Input: part model. Units: mm. Frame: model coordinates. Face numbers are marked on the shaded views. A direction names the side the tool comes from. Coordinates: 2 decimals unless noted, no trailing zeros. Write each loop counter-clockwise with the first axis right and the second up, starting at its lowest first coordinate (ties: lowest second). Pieces come first, ordered by that corner, then holes. Notation, with made-up numbers: (-13.75, -28) -> (34.25, -28) arc R24 cw to (34.25, -11) -> close; hole circle Ø3 at (51, 71). An arc over 180 degrees is marked (long way). Use one line per item in the form item = value. Start each with the question number.
(1) Cut plane A-A on x = 0. Return the cut outline in (y, z).
(2) First-contact query: pin 1 (10 mm diameter, centred on y = 6.5, z = -19, fed in from -X); pin 2 (4 mm diameter, centred on x = -9, y = 0, fed in from +Z); pin 3 (12 mm diameter, centred on x = 6.5, z = -1, fed in from -Y); pin 4 (3 mm diameter, centred on x = -10.5, y = 6, fed in from -Z). Flat tips, straight axial feed; report the tip coordinate or a pass-through.
(3) Pull-direction query (Z, two-part tool) for the marked faces 1, 2 and 3; classes: released by +Z, released by -Z, zero draft, split by the parting line, or undercut.
(4) Ray query, line 1 along Z through (x, y) = (26.5, -7.25); line 2 along X through (y, z) = (-7.45, 0); line 3 along X through (y, z) = (-7, -22.5). Return the intervals inside material, ascending.
(5) Cut plane B-B on z = 0. Return the cut outline in (x, y), plus the area to 3 significant figures.
(6) Set-up query: the marked faces 4, 5, 6, 7 and 8. Return all of +Z, -Z, +X, -X, +Y, -Y with unobstructed straight access to the full face (end or side cutting, diameter ignored); none if empty.
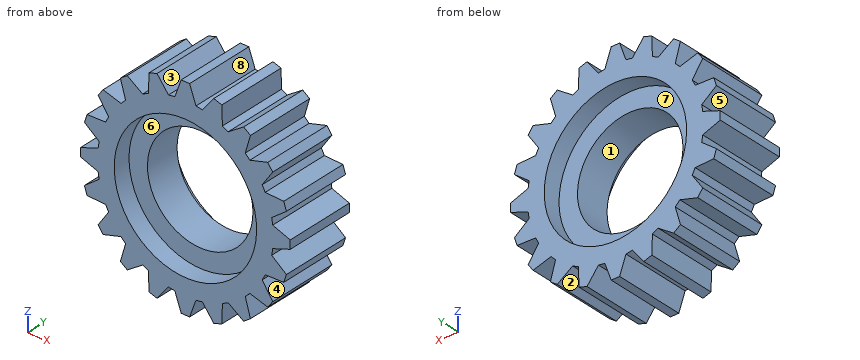
```python
from build123d import *

# Parameters (mm, degrees)
BOSS_EXTRUDE2_START     = -10
BOSS_EXTRUDE2_DEPTH     = 20
CUT_EXTRUDE1_DEPTH      = 5
CUT_EXTRUDE1_DEPTH_BACK = 5
SKETCH3_R               = 15
SKETCH4_R               = 20.25
CUT_EXTRUDE2_DEPTH      = 5


# Read off the part's stored shape, not the designer's step: Boss-Extrude2
with BuildPart() as part:
    # Boss-Extrude2 outline → Boss-Extrude2 (new body)
    with BuildSketch(Plane(origin=(0, 0, 0), x_dir=(1, 0, 0), z_dir=(0, 1, 0)).offset(BOSS_EXTRUDE2_START)):
        with BuildLine():
            Line((24.819347292, -3), (29.819347292, -1.2))
            Line((29.819347292, -1.2), (29.819347292, 1.2))
            Line((29.819347292, 1.2), (24.819347292, 3))
            ThreePointArc((24.819347292, 3), (24.692232517, 3.910710079), (24.531712075, 4.81612943))
            Line((24.531712075, 4.81612943), (28.73075389, 8.073108238))
            Line((28.73075389, 8.073108238), (27.989113104, 10.355643877))
            Line((27.989113104, 10.355643877), (22.677695772, 10.522457624))
            ThreePointArc((22.677695772, 10.522457624), (22.275365258, 11.349365736), (21.842895395, 12.160917759))
            Line((21.842895395, 12.160917759), (24.829892006, 16.555964393))
            Line((24.829892006, 16.555964393), (23.419207401, 18.497605179))
            Line((23.419207401, 18.497605179), (18.316388565, 17.014990742))
            ThreePointArc((18.316388565, 17.014990742), (17.678159939, 17.677179107), (17.016006986, 18.315444473))
            Line((17.016006986, 18.315444473), (18.498605179, 23.418207401))
            Line((18.498605179, 23.418207401), (16.556964393, 24.828892006))
            Line((16.556964393, 24.828892006), (12.162276227, 21.84213902))
            ThreePointArc((12.162276227, 21.84213902), (11.350541159, 22.274766338), (10.523440542, 22.677239672))
            Line((10.523440542, 22.677239672), (10.356643877, 27.988113104))
            Line((10.356643877, 27.988113104), (8.074108238, 28.72975389))
            Line((8.074108238, 28.72975389), (4.817670386, 24.5314095))
            ThreePointArc((4.817670386, 24.5314095), (3.911818446, 24.69205695), (3.00066912, 24.819266404))
            Line((3.00066912, 24.819266404), (1.201, 29.818347292))
            Line((1.201, 29.818347292), (-1.199, 29.818347292))
            Line((-1.199, 29.818347292), (-2.998578144, 24.819519115))
            ThreePointArc((-2.998578144, 24.819519115), (-3.909904803, 24.692360042), (-4.815934726, 24.531750299))
            Line((-4.815934726, 24.531750299), (-8.072108238, 28.72975389))
            Line((-8.072108238, 28.72975389), (-10.354643877, 27.988113104))
            Line((-10.354643877, 27.988113104), (-10.521410966, 22.678181393))
            ThreePointArc((-10.521410966, 22.678181393), (-11.348983821, 22.275559841), (-12.16117688, 21.842751129))
            Line((-12.16117688, 21.842751129), (-16.554964393, 24.828892006))
            Line((-16.554964393, 24.828892006), (-18.496605179, 23.418207401))
            Line((-18.496605179, 23.418207401), (-17.014432073, 18.316907524))
            ThreePointArc((-17.014432073, 18.316907524), (-17.677179115, 17.678159931), (-18.315963478, 17.01544833))
            Line((-18.315963478, 17.01544833), (-23.417207401, 18.497605179))
            Line((-23.417207401, 18.497605179), (-24.827892006, 16.555964393))
            Line((-24.827892006, 16.555964393), (-21.841994742, 12.162535331))
            ThreePointArc((-21.841994742, 12.162535331), (-22.274960948, 11.350159239), (-22.677725349, 10.522393882))
            Line((-22.677725349, 10.522393882), (-27.987113104, 10.355643877))
            Line((-27.987113104, 10.355643877), (-28.72875389, 8.073108238))
            Line((-28.72875389, 8.073108238), (-24.531447735, 4.817475691))
            ThreePointArc((-24.531447735, 4.817475691), (-24.692184512, 3.91101317), (-24.819438268, 2.999247249))
            Line((-24.819438268, 2.999247249), (-29.817347292, 1.2))
            Line((-29.817347292, 1.2), (-29.817347292, -1.2))
            Line((-29.817347292, -1.2), (-24.819438268, -2.999247249))
            ThreePointArc((-24.819438268, -2.999247249), (-24.692184512, -3.91101317), (-24.531447735, -4.817475691))
            Line((-24.531447735, -4.817475691), (-28.72875389, -8.073108238))
            Line((-28.72875389, -8.073108238), (-27.987113104, -10.355643877))
            Line((-27.987113104, -10.355643877), (-22.677725349, -10.522393882))
            ThreePointArc((-22.677725349, -10.522393882), (-22.274960948, -11.350159239), (-21.841994742, -12.162535331))
            Line((-21.841994742, -12.162535331), (-24.827892006, -16.555964393))
            Line((-24.827892006, -16.555964393), (-23.417207401, -18.497605179))
            Line((-23.417207401, -18.497605179), (-18.315963478, -17.01544833))
            ThreePointArc((-18.315963478, -17.01544833), (-17.677179115, -17.678159931), (-17.014432073, -18.316907524))
            Line((-17.014432073, -18.316907524), (-18.496605179, -23.418207401))
            Line((-18.496605179, -23.418207401), (-16.554964393, -24.828892006))
            Line((-16.554964393, -24.828892006), (-12.16117688, -21.842751129))
            ThreePointArc((-12.16117688, -21.842751129), (-11.348983821, -22.275559841), (-10.521410966, -22.678181393))
            Line((-10.521410966, -22.678181393), (-10.354643877, -27.988113104))
            Line((-10.354643877, -27.988113104), (-8.072108238, -28.72975389))
            Line((-8.072108238, -28.72975389), (-4.815934726, -24.531750299))
            ThreePointArc((-4.815934726, -24.531750299), (-3.909904803, -24.692360042), (-2.998578144, -24.819519115))
            Line((-2.998578144, -24.819519115), (-1.199, -29.818347292))
            Line((-1.199, -29.818347292), (1.201, -29.818347292))
            Line((1.201, -29.818347292), (3.00066912, -24.819266404))
            ThreePointArc((3.00066912, -24.819266404), (3.911818446, -24.69205695), (4.817670386, -24.5314095))
            Line((4.817670386, -24.5314095), (8.074108238, -28.72975389))
            Line((8.074108238, -28.72975389), (10.356643877, -27.988113104))
            Line((10.356643877, -27.988113104), (10.523440542, -22.677239672))
            ThreePointArc((10.523440542, -22.677239672), (11.350541159, -22.274766338), (12.162276227, -21.84213902))
            Line((12.162276227, -21.84213902), (16.556964393, -24.828892006))
            Line((16.556964393, -24.828892006), (18.498605179, -23.418207401))
            Line((18.498605179, -23.418207401), (17.016006986, -18.315444473))
            ThreePointArc((17.016006986, -18.315444473), (17.678159939, -17.677179107), (18.316388565, -17.014990742))
            Line((18.316388565, -17.014990742), (23.419207401, -18.497605179))
            Line((23.419207401, -18.497605179), (24.829892006, -16.555964393))
            Line((24.829892006, -16.555964393), (21.842895395, -12.160917759))
            ThreePointArc((21.842895395, -12.160917759), (22.275365258, -11.349365736), (22.677695772, -10.522457624))
            Line((22.677695772, -10.522457624), (27.989113104, -10.355643877))
            Line((27.989113104, -10.355643877), (28.73075389, -8.073108238))
            Line((28.73075389, -8.073108238), (24.531712075, -4.81612943))
            ThreePointArc((24.531712075, -4.81612943), (24.692232517, -3.910710079), (24.819347292, -3))
        make_face()
    extrude(amount=BOSS_EXTRUDE2_DEPTH)

    # Sketch3 → Cut-Extrude1 (cut, two sides: drawn at the far end of the back side and taken through both)
    with BuildSketch(Plane(origin=(0, 0, 0), x_dir=(1, 0, 0), z_dir=(0, 1, 0)).offset(-CUT_EXTRUDE1_DEPTH_BACK)):
        with Locations(Location((0, 0, 0), (0, 0, 270))):
            Circle(SKETCH3_R)
    extrude(amount=CUT_EXTRUDE1_DEPTH + CUT_EXTRUDE1_DEPTH_BACK, mode=Mode.SUBTRACT)

    # Sketch4 → Cut-Extrude2 (cut)
    with BuildSketch(Plane(origin=(0, 10, 0), x_dir=(1, 0, 0), z_dir=(0, 1, 0))):
        with Locations(Location((0, 0, 0), (0, 0, 270))):
            Circle(SKETCH4_R)
    cut_extrude2 = extrude(amount=-CUT_EXTRUDE2_DEPTH, mode=Mode.SUBTRACT)

    # Mirror1: Cut-Extrude2 across plane
    add(cut_extrude2.mirror(Plane.ZX), mode=Mode.SUBTRACT)


solid = part.part
```
Values:
q1.outline = (-10, -29.82) -> (10, -29.82) -> (10, -20.25) -> (5, -20.25) -> (5, -15) -> (-5, -15) -> (-5, -20.25) -> (-10, -20.25) -> close; (-10, 20.25) -> (-5, 20.25) -> (-5, 15) -> (5, 15) -> (5, 20.25) -> (10, 20.25) -> (10, 29.82) -> (-10, 29.82) -> close
q2.pin_1 = -24.83
q2.pin_2 = 28.73
q2.pin_3 = through
q2.pin_4 = -28.43
q3.face_1 = undercut
q3.face_2 = released by -Z
q3.face_3 = released by +Z
q4.line_1 = -10.4 to -6.34, -2.39 to 2.39, 6.34 to 10.4
q4.line_2 = -29.82 to -20.25, 20.25 to 29.82
q4.line_3 = -18.23 to -13.13, -10.9 to 10.9, 13.13 to 18.23
q5.outline = (-29.82, -10) -> (-20.25, -10) -> (-20.25, -5) -> (-15, -5) -> (-15, 5) -> (-20.25, 5) -> (-20.25, 10) -> (-29.82, 10) -> close; (15, -5) -> (20.25, -5) -> (20.25, -10) -> (29.82, -10) -> (29.82, 10) -> (20.25, 10) -> (20.25, 5) -> (15, 5) -> close
q5.area = 488 mm2
q6.face_4 = +X, +Y, -Y
q6.face_5 = -X, +Y, -Y
q6.face_6 = -Y
q6.face_7 = +Y
q6.face_8 = +Z, +Y, -Y
